```python
from build123d import *

# Parameters (mm, degrees)
SKETCH1_R           = 3.175
BOSS_EXTRUDE1_DEPTH = 9.525
SKETCH3_R           = 4.7625
BOSS_EXTRUDE2_DEPTH = 6.35
CUT_EXTRUDE1_START  = -6.35
CUT_EXTRUDE1_DEPTH  = 3.571875
CHAMFER1_SIZE       = 0.39624


with BuildPart() as part:
    # Sketch1 → Boss-Extrude1 (new body)
    with BuildSketch(Plane.XY):
        with Locations(Location((0, 0, 0), (0, 0, 180))):
            Circle(SKETCH1_R)
    extrude(amount=BOSS_EXTRUDE1_DEPTH)

    # Sketch2 → Cut-Revolve1 (revolve, cut)
    with BuildSketch(Plane(origin=(0, 0, 0), x_dir=(0, 0, -1), z_dir=(1, 0, 0)), mode=Mode.PRIVATE) as cut_revolve1_sk:
        Polygon((-9.525, 3.175), (-9.525, 2.405444262), (-8.986151271, 3.175), align=None)
    revolve(cut_revolve1_sk.sketch.rotate(Axis((0, 0, 0), (0, 0, 1)), 90), axis=Axis((0, 0, 0), (0, 0, 1)), mode=Mode.SUBTRACT)

    # Sketch3 → Boss-Extrude2 (add)
    with BuildSketch(Plane.XY):
        Circle(SKETCH3_R)
    extrude(amount=-BOSS_EXTRUDE2_DEPTH)

    # Sketch4 → Cut-Extrude1 (cut)
    with BuildSketch(Plane.XY.offset(CUT_EXTRUDE1_START)):
        Polygon((0, -2.749630657), (2.38125, -1.374815329), (2.38125, 1.374815329), (0, 2.749630657), (-2.38125, 1.374815329), (-2.38125, -1.374815329), align=None)
    extrude(amount=CUT_EXTRUDE1_DEPTH, mode=Mode.SUBTRACT)

    # Cut-Extrude2 cone 1 section (through the dimple's axis) → Cut-Extrude2 (revolve, cut)
    with BuildSketch(Plane(origin=(0, 0, -6.35), x_dir=(0, 1, 0), z_dir=(1, 0, 0))):
        Polygon((0, 0), (2.749630657, 0), (0, 2.749630657), align=None)
    revolve(axis=Axis((0, 0, -6.35), (0, 0, 1)), mode=Mode.SUBTRACT)

    # Chamfer1
    chamfer1_edges = [part.edges().sort_by_distance(p)[0] for p in [
        (-4.7625, 0, -6.35),
        (-4.7625, 0, 0),
    ]]
    chamfer(chamfer1_edges, length=CHAMFER1_SIZE)


solid = part.part
```
Here's how the part is built. I have some questions about the finished solid (model axes, mm). A direction names the side the tool comes from. Give positions to 0.01 mm unless a question says otherwise; leave off trailing zeros. Loops run counter-clockwise (first coordinate to the right, second up) from the corner with the lowest first, then second, coordinate; pieces in that order, holes last. Notation, with made-up numbers: M -12.5,16 L 28.5,16 A20 ccw 28.5,53 Z; hole C -17.75,-32 d7. An arc over 180 degrees is marked long. Return JSON: item names as keys, results as strings.
Item 1: I'm going to push flat-ended pins straight in: pin 1 Ø5 at (y, z) = (2, 2) entering from -X; pin 2 Ø2.5 at (x, y) = (0.5, 0) entering from -Z; pin 3 Ø1 at (x, y) = (-3, -0.5) entering from +Z. Where does each tip first touch, or does it pass through?
A:
{"pin 1": "stops at x = -4.59", "pin 2": "stops at z = -2.78", "pin 3": "stops at z = 9.43"}
Item 2: On a 3-axis mill with a long thin cutter (end or side, diameter ignored), from which of +Z, -Z, +X, -X, +Y, -Y can I reach the whole of each face in a straight line? I mean faces 1 (the flat face through (-2, -3, 0)), 2 (the flat face through (0, -3, -6.35)), 3 (the flat face through (0, 0, -2.778)). Say none if no direction works.
A:
{"face 1": "+Z", "face 2": "-Z, +X, -X, +Y, -Y", "face 3": "-Z"}
Item 3: Imagine slicing it at B-B on z = 0.5. List the corners of the cut face in (x, y) for me (3 decimals), then the cut area to 3 significant figures.
A:
{"outline": "C 0,0 d6.35", "area": "31.7 mm^2"}
Item 4: Please list where these lines run through material, in increasing order: line 1 (Z direction, x = 0.75, y = 3.5); line 2 (X direction, y = -1.75, z = -4.25); line 3 (X direction, y = -2, z = -3.75).
A:
{"line 1": "z = -6.35 to 0", "line 2": "x = -4.43 to -1.73, 1.73 to 4.43", "line 3": "x = -4.32 to -1.3, 1.3 to 4.32"}
Item 5: Thinking about a two-plate mould opening in X: for faces 4 (the flat face through (2.381, 0, -5)), 5 (the cylindrical face through (-3.78, -2.9, -3.14)), 6 (the flat face through (0, 0, 9.525)), which applies, released by +X, released by -X, zero draft, split by the parting line, or undercut?
A:
{"face 4": "undercut", "face 5": "split by the parting line", "face 6": "zero draft"}
